from build123d import *

# Parameters (mm, degrees)
SKETCH1_W           = 700
SKETCH1_H           = 100
BOSS_EXTRUDE1_DEPTH = 3
SKETCH11_W          = 14
SKETCH11_H          = 3
CUT_EXTRUDE8_DEPTH  = 10
SKETCH12_W          = 54
SKETCH12_H          = 3
CUT_EXTRUDE9_DEPTH  = 10
SKETCH13_W          = 13
SKETCH13_H          = 3
CUT_EXTRUDE10_DEPTH = 10
SKETCH14_W          = 54
SKETCH14_H          = 3
CUT_EXTRUDE11_DEPTH = 10
SKETCH15_W          = 14
SKETCH15_H          = 3
CUT_EXTRUDE12_DEPTH = 10
SKETCH16_W          = 54
SKETCH16_H          = 3
CUT_EXTRUDE13_DEPTH = 10
SKETCH17_W          = 13
SKETCH17_H          = 3
CUT_EXTRUDE14_DEPTH = 10
SKETCH18_W          = 54
SKETCH18_H          = 3
CUT_EXTRUDE15_DEPTH = 10
SKETCH21_W          = 505
SKETCH21_H          = 3
CUT_EXTRUDE16_DEPTH = 3


with BuildPart() as part:
    # Sketch1 → Boss-Extrude1 (new body)
    with BuildSketch(Plane.XY):
        with Locations((350, 50)):
            Rectangle(SKETCH1_W, SKETCH1_H)
    extrude(amount=BOSS_EXTRUDE1_DEPTH)

    # Sketch11 → Cut-Extrude8 (cut)
    with BuildSketch(Plane(origin=(0, 0, 0), x_dir=(-1, 0, 0), z_dir=(0, 0, -1))):
        with Locations((-693, 1.5)):
            Rectangle(SKETCH11_W, SKETCH11_H)
    extrude(amount=-CUT_EXTRUDE8_DEPTH, mode=Mode.SUBTRACT)

    # Sketch12 → Cut-Extrude9 (cut)
    with BuildSketch(Plane(origin=(0, 0, 0), x_dir=(-1, 0, 0), z_dir=(0, 0, -1))):
        with Locations((-629, 1.5)):
            Rectangle(SKETCH12_W, SKETCH12_H)
    extrude(amount=-CUT_EXTRUDE9_DEPTH, mode=Mode.SUBTRACT)

    # Sketch13 → Cut-Extrude10 (cut)
    with BuildSketch(Plane(origin=(0, 0, 0), x_dir=(-1, 0, 0), z_dir=(0, 0, -1))):
        with Locations((-6.5, 1.5)):
            Rectangle(SKETCH13_W, SKETCH13_H)
    extrude(amount=-CUT_EXTRUDE10_DEPTH, mode=Mode.SUBTRACT)

    # Sketch14 → Cut-Extrude11 (cut)
    with BuildSketch(Plane(origin=(0, 0, 0), x_dir=(-1, 0, 0), z_dir=(0, 0, -1))):
        with Locations((-70, 1.5)):
            Rectangle(SKETCH14_W, SKETCH14_H)
    extrude(amount=-CUT_EXTRUDE11_DEPTH, mode=Mode.SUBTRACT)

    # Sketch15 → Cut-Extrude12 (cut)
    with BuildSketch(Plane(origin=(0, 0, 0), x_dir=(-1, 0, 0), z_dir=(0, 0, -1))):
        with Locations((-693, 98.5)):
            Rectangle(SKETCH15_W, SKETCH15_H)
    extrude(amount=-CUT_EXTRUDE12_DEPTH, mode=Mode.SUBTRACT)

    # Sketch16 → Cut-Extrude13 (cut)
    with BuildSketch(Plane(origin=(0, 0, 0), x_dir=(-1, 0, 0), z_dir=(0, 0, -1))):
        with Locations((-629, 98.5)):
            Rectangle(SKETCH16_W, SKETCH16_H)
    extrude(amount=-CUT_EXTRUDE13_DEPTH, mode=Mode.SUBTRACT)

    # Sketch17 → Cut-Extrude14 (cut)
    with BuildSketch(Plane(origin=(0, 0, 0), x_dir=(-1, 0, 0), z_dir=(0, 0, -1))):
        with Locations((-6.5, 98.5)):
            Rectangle(SKETCH17_W, SKETCH17_H)
    extrude(amount=-CUT_EXTRUDE14_DEPTH, mode=Mode.SUBTRACT)

    # Sketch18 → Cut-Extrude15 (cut)
    with BuildSketch(Plane(origin=(0, 0, 0), x_dir=(-1, 0, 0), z_dir=(0, 0, -1))):
        with Locations((-70, 98.5)):
            Rectangle(SKETCH18_W, SKETCH18_H)
    extrude(amount=-CUT_EXTRUDE15_DEPTH, mode=Mode.SUBTRACT)

    # Sketch21 → Cut-Extrude16 (cut)
    with BuildSketch(Plane.XY.offset(3)):
        with Locations((349.5, 98.5)):
            Rectangle(SKETCH21_W, SKETCH21_H)
    extrude(amount=-CUT_EXTRUDE16_DEPTH, mode=Mode.SUBTRACT)


solid = part.part
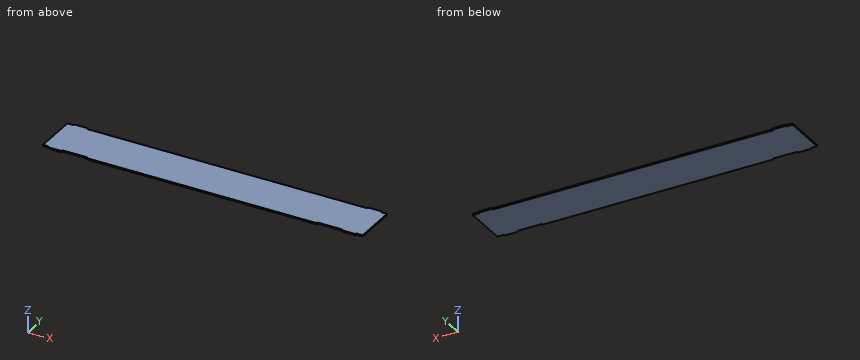
Geometry: final body of the model. Coordinates: model frame, mm. Round coordinates to 2 decimals unless told otherwise and drop trailing zeros. Loops run counter-clockwise (first coordinate to the right, second up) from the corner with the lowest first, then second, coordinate; pieces in that order, holes last. Notation, with made-up numbers: (40, 16) - (99, 16) arc R21 ccw to (99, 53) - close; hole circle Ø10 at (-33, 55.25). An arc over 180 degrees is marked (long way). Write each question's results on one line, items separated by ' | '. Start each with the question number.
1) Line query: probe 1 along Y at (x, z) = (169.5, 1.05). Output: solid intervals per line, ascending. Write a range as [from, to].
2) Cut plane C-C on x = 414. Return loops of the section in (y, z).
3) Cut plane B-B on x = 62.5. Return loops of the section in (y, z), then the cut area to 3 significant figures.
4) Cut plane A-A on z = 2.5. Return loops of the section in (x, y).
5) First-contact query: P1, Ø1, axis at x = 211, z = 2.5, coming from the +Y side; P2, Ø0.9, axis at x = 642, z = 1, coming from the -Y side; P3, Ø0.9, axis at y = 98.5, z = 2, coming from the -X side. Flat tips, straight axial feed; report the tip coordinate or a pass-through.
Verdict:
1) probe 1: y = [0, 97]
2) outline: (0, 0) - (97, 0) - (97, 3) - (0, 3) - close
3) outline: (3, 0) - (97, 0) - (97, 3) - (3, 3) - close | area: 282 mm2
4) outline: (0, 3) - (13, 3) - (13, 0) - (43, 0) - (43, 3) - (97, 3) - (97, 0) - (602, 0) - (602, 3) - (656, 3) - (656, 0) - (686, 0) - (686, 3) - (700, 3) - (700, 97) - (686, 97) - (686, 100) - (656, 100) - (656, 97) - (43, 97) - (43, 100) - (13, 100) - (13, 97) - (0, 97) - close
5) P1: stops at y = 97 | P2: stops at y = 3 | P3: stops at x = 13
